Could you check a few things on this drawing? It's one solid part, dimensions in mm from its lowest x, y, z. Give positions to 0.01 mm unless a question says otherwise; leave off trailing zeros. Order: outer loops, then holes, each group sorted by start corner. A loop starts at its lowest first (then second) coordinate and runs counter-clockwise, first axis right, second up. Notation, with made-up numbers: M 46.5,7 L 76.5,7 A14 cw 76.5,25 Z; hole C 17.25,55 d1. An arc over 180 degrees is marked long. One line per item, written item: value. Start each with the question number.
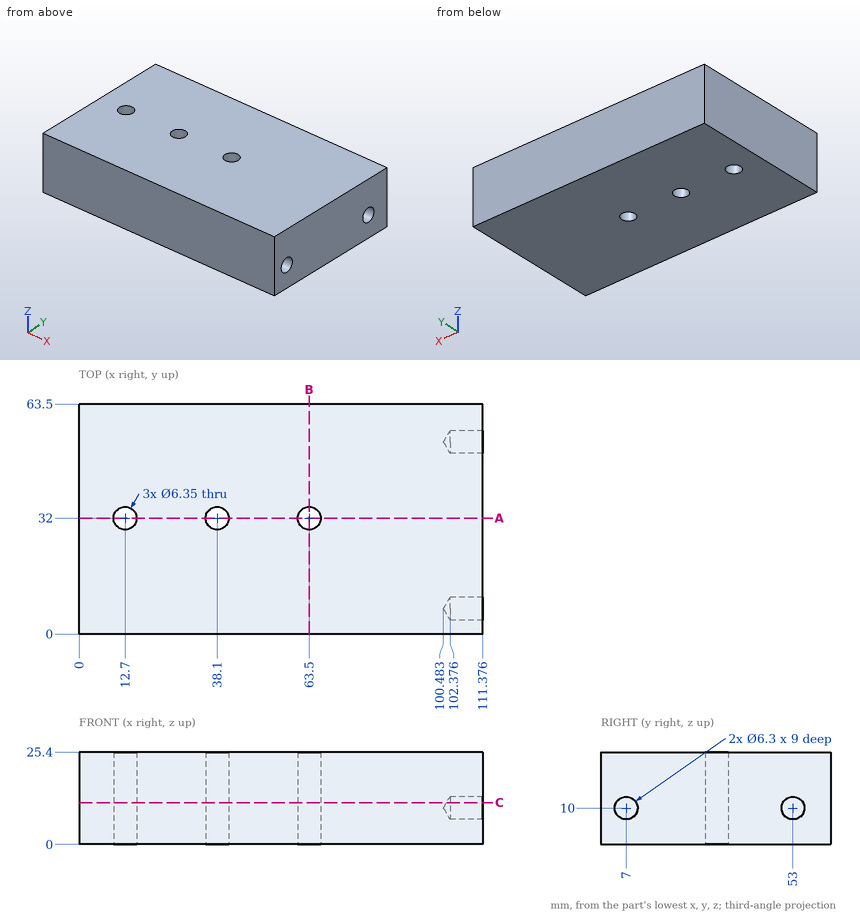
Item 1: Please list where these lines run through material, in increasing order: probe 1 along Y at (x, z) = (12.7, 9) (3 decimals); probe 2 along Z at (x, y) = (108, 53); probe 3 along X at (y, z) = (8.5, 9.75). Write a range as [from, to].
Item 2: Will these pins go through, and if not, where does the flat tip stop? P1, Ø5, axis at y = 7, z = 10, coming from the +X side (1 decimal); P2, Ø4, axis at x = 38.1, y = 32, coming from the -Z side; P3, Ø7, axis at y = 53, z = 10, coming from the +X side.
Item 3: I want a section at B-B on x = 63.5. Write out the boundary of the cut face in (y, z) (3 decimals).
Item 4: I want a section at C-C on z = 11.5. Count the separate pieces of the cut face and the enclosed holes in it, plus the area to 3 significant figures.
Item 5: I want a section at A-A on y = 32. Write out the boundary of the cut face in (x, z) (1 decimal).
Answer below:
1. probe 1: y = [0, 28.825], [35.175, 63.5]
1. probe 2: z = [0, 6.85], [13.15, 25.4]
1. probe 3: x = [0, 101.4]
2. P1: stops at x = 102
2. P2: passes through
2. P3: stops at x = 111.38
3. outline: M 0,0 L 28.825,0 L 28.825,25.4 L 0,25.4 Z; M 35.175,0 L 63.5,0 L 63.5,25.4 L 35.175,25.4 Z
4. separate pieces: 1
4. enclosed holes: 3
4. area: 6,870 mm²
5. outline: M 0,0 L 9.5,0 L 9.5,25.4 L 0,25.4 Z; M 15.9,0 L 34.9,0 L 34.9,25.4 L 15.9,25.4 Z; M 41.3,0 L 60.3,0 L 60.3,25.4 L 41.3,25.4 Z; M 66.7,0 L 111.4,0 L 111.4,25.4 L 66.7,25.4 Z
